from build123d import *

# Parameters (mm, degrees)
SKETCH_1_R          = 10
SKETCH_1_R_2        = 1.75
EXTRUDE_1_DEPTH     = 3
EXTRUDE_2_DEPTH     = 3
SKETCH_7_W          = 35
SKETCH_7_H          = 8
EXTRUDE_3_DEPTH     = 4
FILLET_1_R          = 6
SKETCH_8_R          = 1.75
CUT_EXTRUDE_2_DEPTH = 8
FILLET_2_R          = 2
SKETCH_10_R         = 2.05
CUT_EXTRUDE_3_DEPTH = 6


with BuildPart() as part:
    # Эскиз1 → Бобышка-Вытянуть1 (new body)
    with BuildSketch(Plane.XY):
        Circle(SKETCH_1_R)
        with Locations((-7, 0)):
            Circle(SKETCH_1_R_2, mode=Mode.SUBTRACT)
        with Locations((0, 7)):
            Circle(SKETCH_1_R_2, mode=Mode.SUBTRACT)
        with Locations((7, 0)):
            Circle(SKETCH_1_R_2, mode=Mode.SUBTRACT)
        with Locations((0, -7)):
            Circle(SKETCH_1_R_2, mode=Mode.SUBTRACT)
    extrude(amount=EXTRUDE_1_DEPTH)

    # Эскиз6 → Бобышка-Вытянуть2 (add)
    with BuildSketch(Plane.XY.offset(3)):
        with BuildLine():
            Line((-7.5, 15), (-7.5, 6.614378278))
            ThreePointArc((-7.5, 6.614378278), (0, 10), (7.5, 6.614378278))
            Line((7.5, 6.614378278), (7.5, 15))
            Line((7.5, 15), (17.5, 15))
            Line((17.5, 15), (17.5, 23))
            Line((17.5, 23), (-17.5, 23))
            Line((-17.5, 23), (-17.5, 15))
            Line((-17.5, 15), (-7.5, 15))
        make_face()
    extrude(amount=-EXTRUDE_2_DEPTH)

    # Эскиз7 → Бобышка-Вытянуть3 (add)
    with BuildSketch(Plane.XY.offset(3)):
        with Locations((0, 19)):
            Rectangle(SKETCH_7_W, SKETCH_7_H)
    extrude(amount=EXTRUDE_3_DEPTH)

    # Скругление1
    fillet_1_edges = [part.edges().sort_by_distance(p)[0] for p in [
        (-7.5, 15, 1.5),
        (7.5, 15, 1.5),
    ]]
    fillet(fillet_1_edges, radius=FILLET_1_R)

    # Эскиз8 → Вырез-Вытянуть2 (cut, through all)
    with BuildSketch(Plane.XY.offset(7)):
        with Locations((0, 19)):
            Circle(SKETCH_8_R)
        with Locations((-14, 19)):
            Circle(SKETCH_8_R)
        with Locations((14, 19)):
            Circle(SKETCH_8_R)
    extrude(amount=-CUT_EXTRUDE_2_DEPTH, mode=Mode.SUBTRACT)

    # Скругление2
    fillet_2_edges = [part.edges().sort_by_distance(p)[0] for p in [
        (-17.5, 15, 3.5),
        (-17.5, 23, 3.5),
        (17.5, 23, 3.5),
        (17.5, 15, 3.5),
    ]]
    fillet(fillet_2_edges, radius=FILLET_2_R)

    # Эскиз10 → Вырез-Вытянуть3 (cut)
    with BuildSketch(Plane.XY.offset(7)):
        with Locations((-14, 19)):
            Circle(SKETCH_10_R)
        with Locations((0, 19)):
            Circle(SKETCH_10_R)
        with Locations((14, 19)):
            Circle(SKETCH_10_R)
    extrude(amount=-CUT_EXTRUDE_3_DEPTH, mode=Mode.SUBTRACT)


solid = part.part
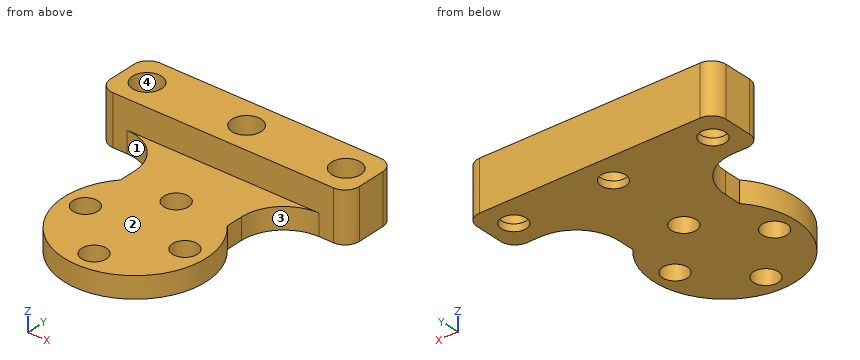
Input: part model. Units: mm. Frame: model coordinates. Face numbers are marked on the shaded views. A direction names the side the tool comes from. Round coordinates to 2 decimals unless told otherwise and drop trailing zeros. Loops run counter-clockwise (first coordinate to the right, second up) from the corner with the lowest first, then second, coordinate; pieces in that order, holes last. Notation, with made-up numbers: (-19, 67.25) -> (26, 67.25) arc R26 ccw to (26, 95.25) -> close; hole circle Ø1 at (57.25, 25). An arc over 180 degrees is marked (long way). Answer as a JSON object with one key per item and string values. Group by question number.
1) Section query C-C on z = 3.75. Output: boundary loops of the cut face in (x, y).
2) Ray query, L1, parallel to Y at x = 0, z = 1.8; L2, parallel to Y at x = -14, z = 0.7; L3, parallel to Y at x = 0, z = 4. Return the intervals inside material, ascending.
3) Pin query (flat end, axial travel): pin 1 (1.9 mm diameter, centred on y = 8, z = 1.5, fed in from +X); pin 2 (4 mm diameter, centred on x = -3.5, z = 2.5, fed in from -Y); pin 3 (2 mm diameter, centred on x = 14, y = 19, fed in from +Z); pin 4 (1.2 mm diameter, centred on y = 8, z = 1, fed in from -X). Return the tip coordinate at first contact, or that it passes through.
4) Section query B-B on x = 0. Output: boundary loops of the cut face in (y, z), plus the area to 3 significant figures.
5) Reachability of the marked faces 1, 2, 3 and 4 from +Z, -Z, +X, -X, +Y, -Y: full face, straight path, thin tool, end or side. Return the list, or none.
6) Section query A-A on y = 0. Output: boundary loops of the cut face in (x, z), plus the area to 3 significant figures.
7) Section query D-D on y = 19. Output: boundary loops of the cut face in (x, z), plus the area to 3 significant figures.
Reply:
{
 "1": {"outline": "(-17.5, 17) arc R2 ccw to (-15.5, 15) -> (15.5, 15) arc R2 ccw to (17.5, 17) -> (17.5, 21) arc R2 ccw to (15.5, 23) -> (-15.5, 23) arc R2 ccw to (-17.5, 21) -> close; hole circle Ø4.1 at (-14, 19); hole circle Ø4.1 at (0, 19); hole circle Ø4.1 at (14, 19)"},
 "2": {"L1": "y = -10 to -8.75, -5.25 to 5.25, 8.75 to 16.95, 21.05 to 23", "L2": "y = 15 to 17.25, 20.75 to 23", "L3": "y = 15 to 16.95, 21.05 to 23"},
 "3": {"pin 1": "stops at x = 7.5", "pin 2": "stops at y = -9.89", "pin 3": "passes through", "pin 4": "stops at x = -7.5"},
 "4": {"outline": "(-10, 0) -> (-8.75, 0) -> (-8.75, 3) -> (-10, 3) -> close; (-5.25, 0) -> (5.25, 0) -> (5.25, 3) -> (-5.25, 3) -> close; (8.75, 0) -> (17.25, 0) -> (17.25, 1) -> (16.95, 1) -> (16.95, 7) -> (15, 7) -> (15, 3) -> (8.75, 3) -> close; (20.75, 0) -> (23, 0) -> (23, 7) -> (21.05, 7) -> (21.05, 1) -> (20.75, 1) -> close", "area": "81.9 mm2"},
 "5": {"face 1": "+Z, -Z, -X", "face 2": "+Z, +X, -X, -Y", "face 3": "+Z, -Z, +X", "face 4": "+Z"},
 "6": {"outline": "(-10, 0) -> (-8.75, 0) -> (-8.75, 3) -> (-10, 3) -> close; (-5.25, 0) -> (5.25, 0) -> (5.25, 3) -> (-5.25, 3) -> close; (8.75, 0) -> (10, 0) -> (10, 3) -> (8.75, 3) -> close", "area": "39.0 mm2"},
 "7": {"outline": "(-17.5, 0) -> (-15.75, 0) -> (-15.75, 1) -> (-16.05, 1) -> (-16.05, 7) -> (-17.5, 7) -> close; (-12.25, 0) -> (-1.75, 0) -> (-1.75, 1) -> (-2.05, 1) -> (-2.05, 7) -> (-11.95, 7) -> (-11.95, 1) -> (-12.25, 1) -> close; (1.75, 0) -> (12.25, 0) -> (12.25, 1) -> (11.95, 1) -> (11.95, 7) -> (2.05, 7) -> (2.05, 1) -> (1.75, 1) -> close; (15.75, 0) -> (17.5, 0) -> (17.5, 7) -> (16.05, 7) -> (16.05, 1) -> (15.75, 1) -> close", "area": "161 mm2"}
}
